Can you work these out from the model? Positions are in its coordinate system, mm. A direction names the side the tool comes from. Coordinates: 2 decimals unless noted, no trailing zeros. Loops run counter-clockwise (first coordinate to the right, second up) from the corner with the lowest first, then second, coordinate; pieces in that order, holes last. Notation, with made-up numbers: M -40,81.25 L -30,81.25 A5 ccw -30,89.25 Z; hole C 64.5,27 d3. An arc over 180 degrees is marked long. Answer as a JSON object with one key per item and string values. Group by question number.
Item 1: Suppose I cut it at C-C (x = 70.5). Write out the boundary of the cut face in (y, z) (1 decimal), then the cut area to 3 significant figures.
Item 2: We'd pull the mould along X, two halves only. Please class faces 1 (the flat face through (0, -38, 67)), 2 (the flat face through (141.288, -39, 67)), 3 (the flat face through (144.462, -38, 67)), 4 (the flat face through (73, -1, 134.938)): +X half, -X half, draft (parallel to the pull), parting line (faces both ways), or undercut.
Item 3: Suppose I cut it at A-A (y = -43.5). Write out the boundary of the cut face in (x, z) (1 decimal), then the cut area to 3 significant figures.
Item 4: Which directions (+Z, -Z, +X, -X, +Y, -Y) give clear straight access to the entire face, cutting with the end or side of a thin tool? Please do faces 5 (the flat face through (72, -1, 0)), 6 (the flat face through (3.175, -40, 67)).
Item 5: If I drill on line 1 (X direction, y = -64.5, z = 50.5) (1 decimal); line 2 (Y direction, x = 75, z = 61.5) (3 decimals), over which ranges is the centre line in solid material (lowest first)?
Item 6: I'm going to push flat-ended pins straight in: pin 1 Ø3.5 at (y, z) = (-78.5, 34) entering from -X; pin 2 Ø3.5 at (x, z) = (143, 43.5) entering from -Y (3 decimals); pin 3 Ø1.6 at (x, z) = (1, 96.5) entering from -Y; pin 4 Ø4 at (x, z) = (92, 41) entering from -Y (3 decimals). Where does each tip first touch, or does it pass through?
Autodesk Fusion 360 part; units mm, degrees
sketch "Sketch1" plane through (0, 0, 0) normal (0, 0, 1) x (1, 0, 0)
  line L0 (0, 0) -> (0, -76.2)
  line L1 (0, -76.2) -> (3.175, -76.2)
  line L2 (3.175, -76.2) -> (3.175, -3.175)
  line L3 (0, 0) -> (144.4625, 0)
  line L4 (144.4625, 0) -> (144.4625, -76.2)
  line L5 (144.4625, -76.2) -> (141.2875, -76.2)
  line L6 (141.2875, -76.2) -> (141.2875, -3.175)
  line L7 (141.2875, -3.175) -> (3.175, -3.175)
  dimension "d1" = 76.2
  dimension "d2" = 3.175
  dimension "d3" = 73.025
  dimension "d4" = 144.4625
  dimension "d5" = 76.2
  dimension "d6" = 3.175
  dimension "d7" = 73.025
extrude "Extrude1" add sketch "Sketch1" along normal blind 134.9375
sketch "Sketch2" plane through (141.2875, 0, 0) normal (-1, 0, 0) x (0, -1, 0)
  line L0 (3.175, 0) -> (76.2, 0)
  line L1 (76.2, 0) -> (76.2, 134.9375)
  line L2 (76.2, 134.9375) -> (3.175, 134.9375)
  line L3 (3.175, 134.9375) -> (3.175, 0)
  line L4 (76.2, 134.9375) -> (73.025, 134.9375)
  line L5 (73.025, 134.9375) -> (73.025, 0)
  line L6 (73.025, 0) -> (76.2, 0)
  line L7 (76.2, 0) -> (76.2, 134.9375)
  dimension "d11" = 3.175
revolve "Revolve1" add sketch "Sketch2" angle 90 about axis through (141.2875, -76.2, 0) along (0, 0, 1) contours L0 L1 L2 L4 L5 L6 L7
sketch "Sketch3" plane through (0, -76.2, 0) normal (0, -1, 0) x (1, 0, 0)
  line L0 (138.1125, 0) -> (144.4625, 0)
  line L1 (144.4625, 0) -> (144.4625, 134.9375)
  line L2 (144.4625, 134.9375) -> (138.1125, 134.9375)
  line L3 (138.1125, 134.9375) -> (138.1125, 0)
  line L4 (138.1125, 134.9375) -> (141.2875, 134.9375)
  line L5 (141.2875, 134.9375) -> (141.2875, 0)
  line L6 (141.2875, 0) -> (138.1125, 0)
  line L7 (138.1125, 0) -> (138.1125, 134.9375)
  dimension "d13" = 3.175
extrude "Extrude2" add sketch "Sketch3" along normal blind 3.175 contours L0 L2 L3 L4 L5 L6 L7
equation "Length = ( 10.625 / 2 ) * 1 in"
equation "d9 = Length"
From the geometry:
{
 "1": {"outline": "M -3.2,0 L 0,0 L 0,134.9 L -3.2,134.9 Z", "area": "428 mm2"},
 "2": {"face 1": "-X half", "face 2": "undercut", "face 3": "+X half", "face 4": "draft"},
 "3": {"outline": "M 0,0 L 3.2,0 L 3.2,134.9 L 0,134.9 Z; M 141.3,0 L 144.5,0 L 144.5,134.9 L 141.3,134.9 Z", "area": "857 mm2"},
 "4": {"face 5": "-Z, +X, -X, +Y, -Y", "face 6": "+Z, -Z, -Y"},
 "5": {"line 1": "0 to 3.2, 141.3 to 144.5", "line 2": "-3.175 to 0"},
 "6": {"pin 1": "x = 138.11", "pin 2": "y = -79.375", "pin 3": "y = -76.2", "pin 4": "y = -3.175"}
}
